```python
from build123d import *

# Parameters (mm, degrees)
EXTRUDE_1_DEPTH     = 9.5
SKETCH_3_R          = 7.5
CUT_EXTRUDE_2_DEPTH = 39.977557645
FILLET_2_R          = 3


with BuildPart() as part:
    # 草图1 → 凸台-拉伸1 (new body)
    with BuildSketch(Plane(origin=(0, 0, 0), x_dir=(1, 0, 0), z_dir=(0, 1, 0))):
        Polygon((0, 0), (-30, 0), (-30, 23), (-14, 23), (-14, 22.98886809), (14, 22.98886809), (14, 23), (30, 23), (30, 0), align=None)
    extrude(amount=EXTRUDE_1_DEPTH)

    # 草图3 → 切除-拉伸2 (cut, through all)
    with BuildSketch(Plane(origin=(0, 9.5, 0), x_dir=(1, 0, 0), z_dir=(0, 1, 0))):
        with Locations(Location((0, 11.48886809, 0), (0, 0, 270))):
            Circle(SKETCH_3_R)
        with Locations(Location((-20, 9.65, 0), (0, 0, 270))):
            Circle(SKETCH_3_R)
        with Locations(Location((20, 9.65, 0), (0, 0, 270))):
            Circle(SKETCH_3_R)
    extrude(amount=-CUT_EXTRUDE_2_DEPTH, mode=Mode.SUBTRACT)

    # 圆角2
    # the kernel refuses this fillet: 3 mm, written as the material it adds along each edge
    with BuildSketch(Plane(origin=(14, 0, -22.98886809), x_dir=(0, 0, -1), z_dir=(0, 1, 0))) as fillet_2_piece_1:
        with BuildLine():
            CenterArc((3, 0.25820058), FILLET_2_R, 180, 4.937376285)
            Line((0, 0.25820058), (0, 0))
            Line((0, 0), (0.01113191, 0))
        make_face()
    extrude(amount=9.5)
    with BuildSketch(Plane(origin=(-14, 0, -22.98886809), x_dir=(0, 0, -1), z_dir=(0, 1, 0))) as fillet_2_piece_2:
        with BuildLine():
            CenterArc((3, -0.25820058), FILLET_2_R, 175.062623715, 4.937376285)
            Line((0, -0.25820058), (0, 0))
            Line((0, 0), (0.01113191, 0))
        make_face()
    extrude(amount=9.5)
    # the kernel refuses this fillet: 3 mm, written as the material it takes off along each edge
    with BuildSketch(Plane(origin=(30, -7.5, -23), x_dir=(0, 0, 1), z_dir=(0, 1, 0))) as fillet_2_2_piece_1:
        with BuildLine():
            CenterArc((FILLET_2_R, -FILLET_2_R), FILLET_2_R, 90, 90)
            Line((0, -FILLET_2_R), (0, 0))
            Line((0, 0), (FILLET_2_R, 0))
        make_face()
    extrude(amount=24.5, mode=Mode.SUBTRACT)
    with BuildSketch(Plane(origin=(-30, -7.5, -23), x_dir=(0, 0, 1), z_dir=(0, 1, 0))) as fillet_2_2_piece_2:
        with BuildLine():
            CenterArc((FILLET_2_R, FILLET_2_R), FILLET_2_R, 180, 90)
            Line((0, FILLET_2_R), (0, 0))
            Line((0, 0), (FILLET_2_R, 0))
        make_face()
    extrude(amount=24.5, mode=Mode.SUBTRACT)


solid = part.part
```
Could you check a few things on this model? Use its own coordinates, in mm. Round coordinates to 2 decimals unless told otherwise and drop trailing zeros. Loops run counter-clockwise (first coordinate to the right, second up) from the corner with the lowest first, then second, coordinate; pieces in that order, holes last. Notation, with made-up numbers: (18.25, 72.25) -> (62.25, 72.25) arc R20 cw to (62.25, 88.25) -> close; hole circle Ø5 at (-11, -13). An arc over 180 degrees is marked (long way). Put each result on its own line as item: value.
Q1. I want a section at C-C on z = -13. Write out the boundary of the cut face in (x, y), and give its area (3 significant figures).
Checks:
outline: (-30, 0) -> (-26.71, 0) -> (-26.71, 9.5) -> (-30, 9.5) -> close; (-13.29, 0) -> (-7.35, 0) -> (-7.35, 9.5) -> (-13.29, 9.5) -> close; (7.35, 0) -> (13.29, 0) -> (13.29, 9.5) -> (7.35, 9.5) -> close; (26.71, 0) -> (30, 0) -> (30, 9.5) -> (26.71, 9.5) -> close
area: 175 mm2
Q2. For pin 1 Ø9 at (x, z) = (-20, -9.65) entering from -Y; pin 2 Ø2 at (x, y) = (11.5, 4.5) entering from -Z, each with a flat end and sliding along its axis, tell me the tip position at first contact or that it passes through.
Checks:
pin 1: through
pin 2: z = -22.99
Q3. I want a section at B-B on y = 2.5. Write out the boundary of the cut face in (x, z), and give its area (3 significant figures).
Checks:
outline: (-30, -20) arc R3 ccw to (-27, -23) -> (-14, -23) arc R3 cw to (-13.74, -22.99) -> (13.74, -22.99) arc R3 cw to (14, -23) -> (27, -23) arc R3 ccw to (30, -20) -> (30, 0) -> (-30, 0) -> close; hole circle Ø15 at (-20, -9.65); hole circle Ø15 at (0, -11.49); hole circle Ø15 at (20, -9.65)
area: 846 mm2
Q4. I want a section at D-D on z = -17.75. Write out the boundary of the cut face in (x, y).
Checks:
outline: (-30, 0) -> (-4.13, 0) -> (-4.13, 9.5) -> (-30, 9.5) -> close; (4.13, 0) -> (30, 0) -> (30, 9.5) -> (4.13, 9.5) -> close
Q5. Thinking about a two-plate mould opening in X: for faces 1 (the flat face through (0, 5, 0)), 2 (the cylindrical face through (27.436, 4.816, -10.626)), 3 (the cylindrical face through (-29.1, 4.68, -22.14)), 4 (the cylindrical face through (-2.87, 4.82, -4.56)), which applies, pulls with the +X half, pulls with the -X half, needs draft (parallel to the pull), parting line crosses it, or undercut?
Checks:
face 1: needs draft
face 2: undercut
face 3: pulls with the -X half
face 4: undercut
Q6. I want a section at A-A on x = 0. Write out the boundary of the cut face in (y, z), and give its area (3 significant figures).
Checks:
outline: (0, -22.99) -> (9.5, -22.99) -> (9.5, -18.99) -> (0, -18.99) -> close; (0, -3.99) -> (9.5, -3.99) -> (9.5, 0) -> (0, 0) -> close
area: 75.9 mm2
Q7. Please list where these lines run through material, in increasing order: line 1 (X direction, y = 4.25, z = -9.65); line 2 (X direction, y = 4.25, z = -8.75); line 3 (Z direction, x = 9, y = 1.5). Write a range as from..to.
Checks:
line 1: -30..-27.5, -12.5..-7.27, 7.27..12.5, 27.5..30
line 2: -30..-27.45, -12.55..-6.98, 6.98..12.55, 27.45..30
line 3: -22.99..0
